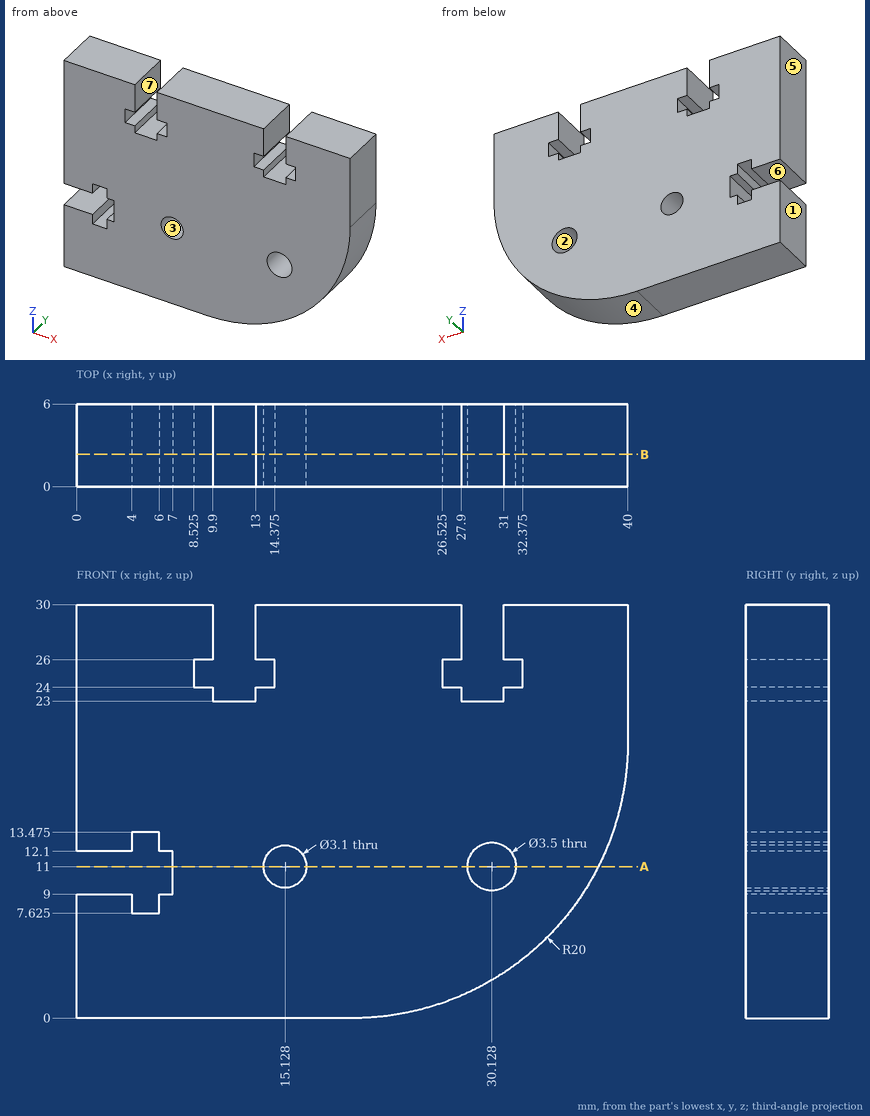
Geometry: see drawing. Coordinates: mm, zero at the bounding-box minimum. A direction names the side the tool comes from. Coordinates: 2 decimals unless noted, no trailing zeros. Loops run counter-clockwise (first coordinate to the right, second up) from the corner with the lowest first, then second, coordinate; pieces in that order, holes last.
(1) Set-up query: the marked faces 5, 6 and 7. Return all of +Z, -Z, +X, -X, +Y, -Y with unobstructed straight access to the full face (end or side cutting, diameter ignored); none if empty.
(2) Section A-A on z = 11. Return the cut outline in (x, y).
(3) First-contact query: pin 1 Ø1 at (x, y) = (34.5, 1) entering from -Z; pin 2 Ø0.7 at (x, y) = (31.5, 3.5) entering from -Z. Flat tips, straight axial feed; report the tip coordinate or a pass-through.
(4) Section B-B on y = 2.35. Count the separate pieces of the cut face and the enclosed holes in it, then the cut area to 3 significant figures.
(5) Material intervals for probe 1 along X at (y, z) = (3.95, 27); probe 2 along X at (y, z) = (1.8, 11.75); probe 3 along Z at (x, y) = (5.5, 2.35) (3 decimals), sorted ascending.
(6) Pull-direction query (Z, two-part tool) for the marked faces 1, 2, 3 and 4; classes: released by +Z, released by -Z, zero draft, split by the parting line, or undercut.
Data:
1. face 5: +Z, -Z, -X, +Y, -Y
1. face 6: -X, +Y, -Y
1. face 7: +Z, +Y, -Y
2. outline: (7, 0) - (13.58, 0) - (13.58, 6) - (7, 6) - close; (16.68, 0) - (28.38, 0) - (28.38, 6) - (16.68, 6) - close; (31.88, 0) - (37.86, 0) - (37.86, 6) - (31.88, 6) - close
3. pin 1: stops at z = 5.72
3. pin 2: stops at z = 3.4
4. separate pieces: 1
4. enclosed holes: 2
4. area: 1,020 mm2
5. probe 1: x = 0 to 9.9, 13 to 27.9, 31 to 40
5. probe 2: x = 7 to 13.77, 16.48 to 28.55, 31.71 to 38.22
5. probe 3: z = 0 to 7.625, 13.475 to 30
6. face 1: zero draft
6. face 2: undercut
6. face 3: undercut
6. face 4: released by -Z
